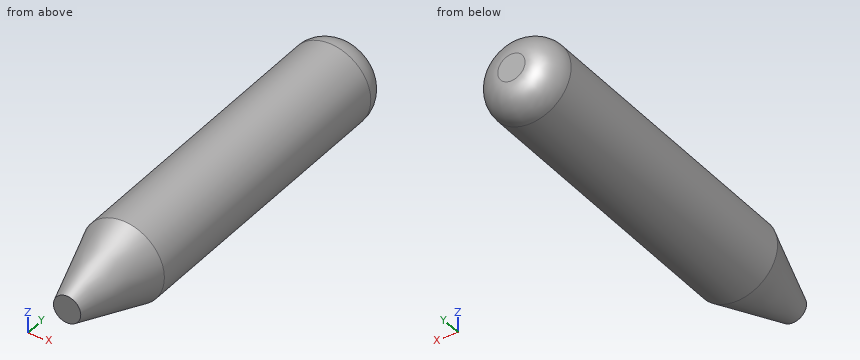
```python
from build123d import *

# Parameters (mm, degrees)
CROQUIS1_R              = 15
SALIENTE_EXTRUIR1_DEPTH = 150
REDONDEO5_R             = 10
CHAFL_N2_SIZE           = 10
CHAFL_N2_SIZE2          = 30


with BuildPart() as part:
    # Croquis1 → Saliente-Extruir1 (new body)
    with BuildSketch(Plane(origin=(0, 0, 0), x_dir=(1, 0, 0), z_dir=(0, 1, 0))):
        with Locations(Location((0, 0, 0), (0, 0, 270))):
            Circle(CROQUIS1_R)
    extrude(amount=SALIENTE_EXTRUIR1_DEPTH)

    # Redondeo5
    redondeo5_edges = [part.edges().sort_by_distance(p)[0] for p in [
        (0, 150, -15),
    ]]
    fillet(redondeo5_edges, radius=REDONDEO5_R)

    # Chaflán2
    chafl_n2_edges = [part.edges().sort_by_distance(p)[0] for p in [
        (0, 0, -15),
    ]]
    chafl_n2_side = [part.faces().sort_by_distance(p)[0] for p in [
        (0, 0, 0),
    ]]
    chamfer(chafl_n2_edges, length=CHAFL_N2_SIZE, length2=CHAFL_N2_SIZE2, reference=chafl_n2_side[0])


solid = part.part
```
CAD build for the part. Positions are in the model's coordinates, mm. Round coordinates to 2 decimals unless told otherwise and drop trailing zeros. Write each loop counter-clockwise with the first axis right and the second up, starting at its lowest first coordinate (ties: lowest second). Pieces come first, ordered by that corner, then holes. Notation, with made-up numbers: M 35,-34.75 L 78,-34.75 A14 ccw 78,-14.75 Z; hole C 4.5,-8 d9. An arc over 180 degrees is marked long. One line per question, with ' | ' between items.
1. Cut at A-A on y = 108.5. Write the cut outline in (x, z), and give its area (3 significant figures).
Working result:
outline: C 0,0 d30 | area: 707 mm2
2. Pin check, flat tips, straight feed: pin 1 Ø4 at (y, z) = (125, 11.5) entering from -X; pin 2 Ø5 at (x, y) = (-4.5, 43.5) entering from +Z; pin 3 Ø5 at (x, y) = (-5.5, 81.5) entering from -Z. Stop position of each tip, or through.
Working result:
pin 1: x = -11.61 | pin 2: z = 14.87 | pin 3: z = -14.7
3. Probe L1, parallel to Z at x = -0.75, y = 46; L2, parallel to Z at x = 3.5, y = 60.5; L3, parallel to X at y = 114.5, z = 6.25. List the from-to ranges inside material, lowest first. Write a range as from..to.
Working result:
L1: -14.98..14.98 | L2: -14.59..14.59 | L3: -13.64..13.64
